Check sheet for the drawn part. Datum: minimum x, y, z corner. Units: mm. Give positions to 0.01 mm unless a question says otherwise; leave off trailing zeros. Loops run counter-clockwise (first coordinate to the right, second up) from the corner with the lowest first, then second, coordinate; pieces in that order, holes last. Notation, with made-up numbers: M 89,70 L 111,70 A13 cw 111,80 Z; hole C 24.25,-10 d10. An arc over 180 degrees is marked long. Write each question's results on one line, items separated by ' | '. Start each with the question number.
1. Sectioned sample at A-A on y = 5.5. Record the cut outline in (x, z), and give its area (3 significant figures).
2. Sectioned sample at B-B on x = 5.5. Record the cut outline in (y, z), and give its area (3 significant figures).
3. Material ranges on line 1 along Z through (x, y) = (5.5, 10.1); line 2 along Y through (x, z) = (5.5, 12.5); line 3 along Y through (x, z) = (7.25, 19), recorded low to high.
4. Draft check along Y on the marked faces 1, 2 and 3. Enter one of: pulls with the +Y half, pulls with the -Y half, needs draft (parallel to the pull), parting line crosses it, or undercut.
5. Go/stop test with flat-tipped pins: pin 1 (4 mm diameter, centred on x = 9.5, z = 12, fed in from -Y); pin 2 (1 mm diameter, centred on y = 2, z = 14.5, fed in from -X); pin 3 (1.1 mm diameter, centred on x = 5.5, z = 3, fed in from +Y); pin 4 (1 mm diameter, centred on y = 2, z = 9.5, fed in from +X). Record where each tip stops, or that it passes through.
6. Sectioned sample at C-C on z = 16.5. Record the cut outline in (x, y), and give its area (3 significant figures).
7. Sectioned sample at D-D on z = 3. Record the cut outline in (x, y).
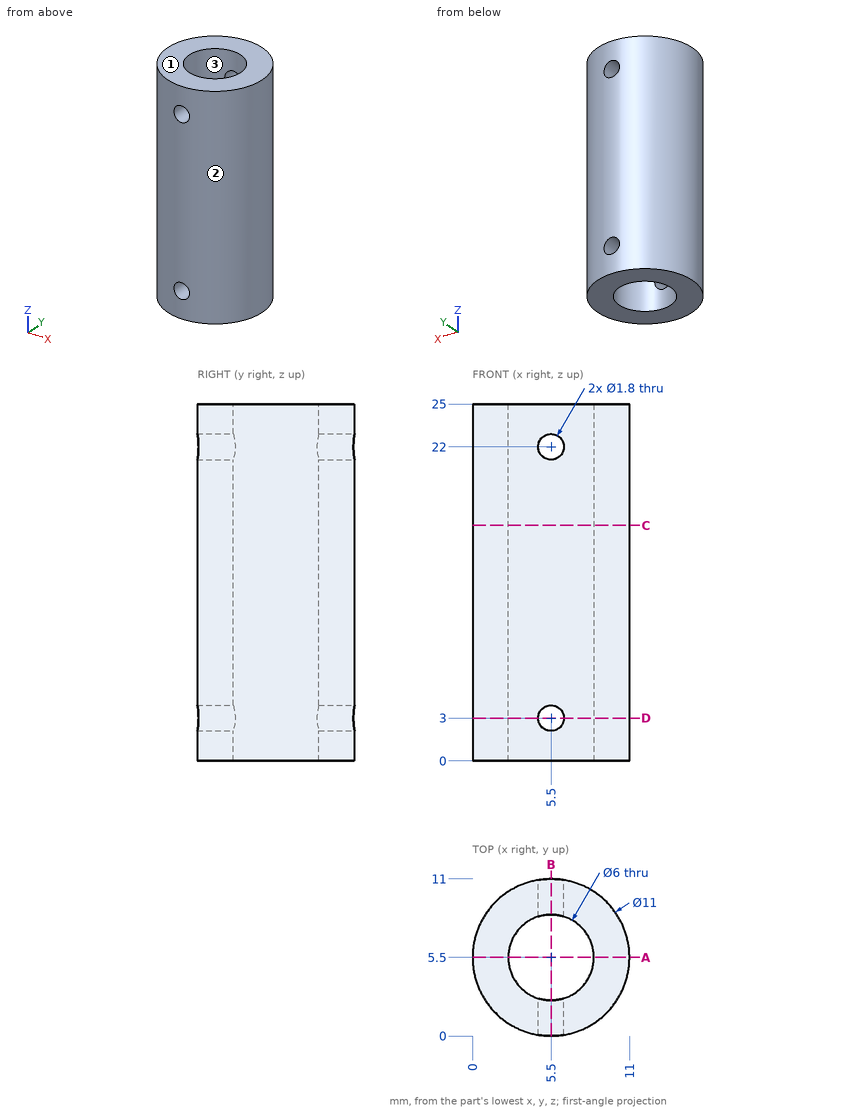
Output values:
1) outline: M 0,0 L 2.5,0 L 2.5,25 L 0,25 Z; M 8.5,0 L 11,0 L 11,25 L 8.5,25 Z | area: 125 mm2
2) outline: M 0,0 L 2.5,0 L 2.5,2.1 L 0,2.1 Z; M 0,3.9 L 2.5,3.9 L 2.5,21.1 L 0,21.1 Z; M 0,22.9 L 2.5,22.9 L 2.5,25 L 0,25 Z; M 8.5,0 L 11,0 L 11,2.1 L 8.5,2.1 Z; M 8.5,3.9 L 11,3.9 L 11,21.1 L 8.5,21.1 Z; M 8.5,22.9 L 11,22.9 L 11,25 L 8.5,25 Z | area: 107 mm2
3) line 1: 0 to 2.1, 3.9 to 21.1, 22.9 to 25 | line 2: 0 to 2.5, 8.5 to 11 | line 3: 0.29 to 3.06, 7.94 to 10.71
4) face 1: needs draft | face 2: parting line crosses it | face 3: undercut
5) pin 1: y = 0.38 | pin 2: x = 0.89 | pin 3: through | pin 4: x = 10.11
6) outline: C 5.5,5.5 d11; hole C 5.5,5.5 d6 | area: 66.8 mm2
7) outline: M 4.6,0.07 L 4.6,2.64 A3 cw 4.6,8.36 L 4.6,10.93 A5.5 ccw Z; M 6.4,0.07 A5.5 ccw 6.4,10.93 L 6.4,8.36 A3 cw 6.4,2.64 Z
